The drawing under review shows one solid part. Ordinate dimensions are in mm from its lowest x, y, z. A direction names the side the tool comes from. Coordinates: 2 decimals unless noted, no trailing zeros. Loops run counter-clockwise (first coordinate to the right, second up) from the corner with the lowest first, then second, coordinate; pieces in that order, holes last. Notation, with made-up numbers: (80.5, 4) - (121.5, 4) arc R14 cw to (121.5, 26) - close; hole circle Ø9 at (20, 1.5). An arc over 180 degrees is marked (long way). Use one line per item in the form item = value. Start each with the question number.
1. Add section B-B on x = 5. Give the boundary of the cut face in (y, z).
2. To check wall thickness, follow probe 1 along X at (y, z) = (16.3, 24.5); probe 2 along X at (y, z) = (19, 15); probe 3 along Y at (x, z) = (6.75, 29.5). State the ranges of each line that lie inside material, in increasing order.
3. Add section D-D on z = 8. Give the boundary of the cut face in (x, y), and give its area (3 significant figures).
4. Add section A-A on z = 24.5. Give the boundary of the cut face in (x, y), and give its area (3 significant figures).
5. For pin 1 Ø1.5 at (y, z) = (17, 12) entering from -X; pin 2 Ø5 at (x, z) = (7, 4.5) entering from +Y; pin 3 Ø6 at (x, y) = (24.5, 12.5) entering from -Z; pin 4 Ø1 at (y, z) = (3.5, 7.5) entering from -X, all flat-tipped, find the tip position at first contact; note any pin that passes through.
6. Machinability: for the marked faces 1, 2, 3 and 4, which of the approach directions +Z, -Z, +X, -X, +Y, -Y give a long, thin tool a straight path to every point of the face, cutting with its end or side? Answer none if there is none.
7. Add section C-C on y = 15.5. Give the boundary of the cut face in (x, z).
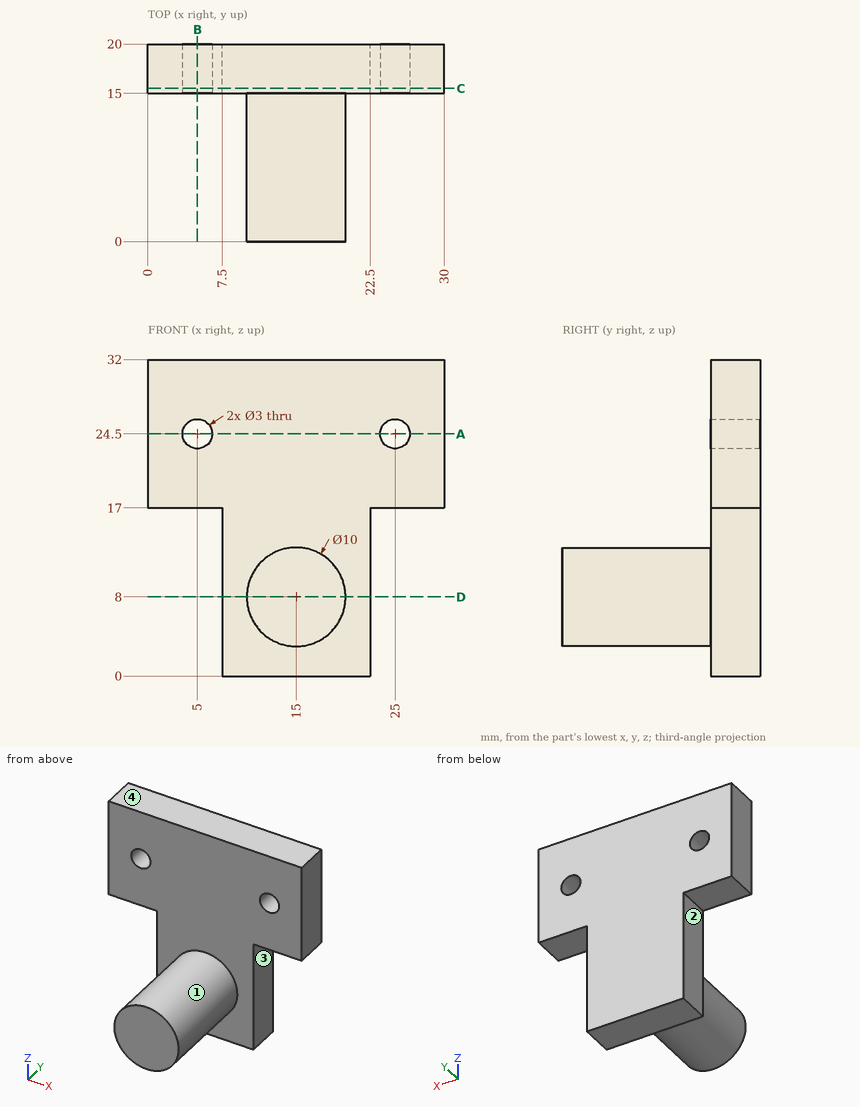
Conclusion:
q1.outline = (15, 17) - (20, 17) - (20, 23) - (15, 23) - close; (15, 26) - (20, 26) - (20, 32) - (15, 32) - close
q2.probe_1 = 0 to 3.5, 6.5 to 23.5, 26.5 to 30
q2.probe_2 = 7.5 to 22.5
q2.probe_3 = 15 to 20
q3.outline = (7.5, 15) - (10, 15) - (10, 0) - (20, 0) - (20, 15) - (22.5, 15) - (22.5, 20) - (7.5, 20) - close
q3.area = 225 mm^2
q4.outline = (0, 15) - (3.5, 15) - (3.5, 20) - (0, 20) - close; (6.5, 15) - (23.5, 15) - (23.5, 20) - (6.5, 20) - close; (26.5, 15) - (30, 15) - (30, 20) - (26.5, 20) - close
q4.area = 120 mm^2
q5.pin_1 = 7.5
q5.pin_2 = 20
q5.pin_3 = 17
q5.pin_4 = 10
q6.face_1 = -Y
q6.face_2 = -Z, -X, +Y, -Y
q6.face_3 = -Z, +X, +Y, -Y
q6.face_4 = +Z, +X, -X, +Y, -Y
q7.outline = (0, 17) - (7.5, 17) - (7.5, 0) - (22.5, 0) - (22.5, 17) - (30, 17) - (30, 32) - (0, 32) - close; hole circle Ø3 at (5, 24.5); hole circle Ø3 at (25, 24.5)
